Work out the finished part from the listing and answer in its coordinate system (mm). Coordinates: 2 decimals unless noted, no trailing zeros. Loops run counter-clockwise (first coordinate to the right, second up) from the corner with the lowest first, then second, coordinate; pieces in that order, holes last.
```python
from build123d import *

# Parameters (mm, degrees)
SKETCH1_R                                = 4.25
BOSS_EXTRUDE1_DEPTH                      = 10
BOSS_EXTRUDE2_START                      = -5
BOSS_EXTRUDE2_DEPTH                      = 15
SKETCH3_W                                = 342
SKETCH3_H                                = 10
BOSS_EXTRUDE3_DEPTH                      = 304
CUT_EXTRUDE1_REACH                       = 381.323
BOSS_EXTRUDE4_DEPTH                      = 3
MIRROR5_AT_THE_SECOND_PLANE_COPY_1_DEPTH = 3


with BuildPart() as part:
    # Sketch1 → Boss-Extrude1 (new body)
    with BuildSketch(Plane(origin=(0, 0, 0), x_dir=(1, 0, 0), z_dir=(0, 1, 0))):
        Polygon((-171, 11.25), (171, 11.25), (171, 0), (171, -13.75), (158, -13.75), (158, 0), (-158, 0), (-158, -13.75), (-171, -13.75), align=None)
        with Locations(Location((-164, 4.25, 0), (0, 0, 270))):
            Circle(SKETCH1_R, mode=Mode.SUBTRACT)
        with Locations(Location((164, 4.25, 0), (0, 0, 90))):
            Circle(SKETCH1_R, mode=Mode.SUBTRACT)
    boss_extrude1 = extrude(amount=BOSS_EXTRUDE1_DEPTH)

    # Sketch2 → Boss-Extrude2 (add)
    with BuildSketch(Plane.XY.offset(13.75).offset(BOSS_EXTRUDE2_START)):
        Polygon((-171, 85), (-171, 0), (-158, 0), (-158, 60), (158, 60), (158, 0), (171, 0), (171, 85), align=None)
    boss_extrude2 = extrude(amount=BOSS_EXTRUDE2_DEPTH)

    # Sketch3 → Boss-Extrude3 (add)
    with BuildSketch(Plane.XY.offset(23.75)):
        with Locations((0, 65)):
            Rectangle(SKETCH3_W, SKETCH3_H)
    extrude(amount=BOSS_EXTRUDE3_DEPTH)

    # Sketch4 → Cut-Extrude1 (cut, up to next)
    with BuildSketch(Plane(origin=(0, 85, 0), x_dir=(1, 0, 0), z_dir=(0, 1, 0)), mode=Mode.PRIVATE) as cut_extrude1_sk1:
        Polygon((-163.5, -23.75), (-5, -23.75), (-5, -327.75), (-163.5, -327.75), (-163.5, -39.75), (-163.5, -34.75), align=None)
    cut_extrude1_tool1 = extrude(cut_extrude1_sk1.sketch, amount=-CUT_EXTRUDE1_REACH, mode=Mode.PRIVATE) & part.part
    # Sketch4 → Cut-Extrude1 (cut, up to next)
    with BuildSketch(Plane(origin=(0, 85, 0), x_dir=(1, 0, 0), z_dir=(0, 1, 0)), mode=Mode.PRIVATE) as cut_extrude1_sk2:
        Polygon((163.5, -23.75), (163.5, -51.4723011), (163.5, -327.75), (5, -327.75), (5, -39.75), (5, -23.75), align=None)
    cut_extrude1_tool2 = extrude(cut_extrude1_sk2.sketch, amount=-CUT_EXTRUDE1_REACH, mode=Mode.PRIVATE) & part.part
    add(cut_extrude1_tool1.solids().sort_by_distance((-84.25, 85, 175.75))[0], mode=Mode.SUBTRACT)
    add(cut_extrude1_tool2.solids().sort_by_distance((84.25, 85, 175.75))[0], mode=Mode.SUBTRACT)

    # Mirror3: Boss-Extrude2 across plane
    add(boss_extrude2.mirror(Plane(origin=(0, 0, 175.75), x_dir=(1, 0, 0), z_dir=(0, 0, -1))))

    # Mirror4: Boss-Extrude1 across plane
    add(boss_extrude1.mirror(Plane(origin=(0, 0, 175.75), x_dir=(1, 0, 0), z_dir=(0, 0, -1))))

    # Sketch7 → Boss-Extrude4 (add)
    with BuildSketch(Plane(origin=(0, 60, 0), x_dir=(-1, 0, 0), z_dir=(0, -1, 0))):
        Polygon((-163.5, -23.75), (-148.5, -23.75), (-163.5, -38.75), align=None)
        Polygon((-5, -23.75), (-20, -23.75), (-5, -38.75), align=None)
    boss_extrude4 = extrude(amount=-BOSS_EXTRUDE4_DEPTH)

    # Mirror5: Boss-Extrude4 across plane
    add(boss_extrude4.mirror(Plane(origin=(0, 0, 175.75), x_dir=(1, 0, 0), z_dir=(0, 0, -1))))

    # Mirror5 at the second plane: Boss-Extrude4 across plane
    add(boss_extrude4.mirror(Plane(origin=(0, 0, 0), x_dir=(0, 0, 1), z_dir=(1, 0, 0))))

    # Mirror5 at the second plane copy 1 sketc → Mirror5 at the second plane copy 1 (add)
    with BuildSketch(Plane(origin=(0, 60, 351.5), x_dir=(1, 0, 0), z_dir=(0, -1, 0))):
        Polygon((-163.5, -23.75), (-148.5, -23.75), (-163.5, -38.75), align=None)
        Polygon((-5, -23.75), (-20, -23.75), (-5, -38.75), align=None)
    extrude(amount=-MIRROR5_AT_THE_SECOND_PLANE_COPY_1_DEPTH)


solid = part.part
```
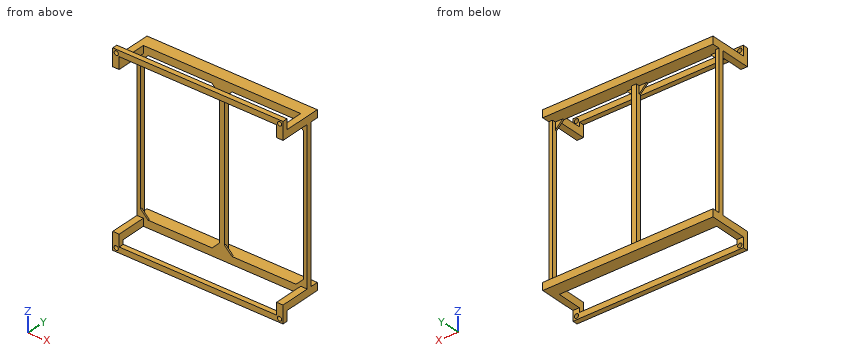
1. A cutting plane is placed at B-B, the plane x = -36.5. Give the vertices of the cut face in (y, z), then the cut area to 3 significant figures.
2. A cutting plane is placed at A-A, the plane z = 47. Give the vertices of the cut face in (x, y), then the cut area to 3 significant figures.
3. Straight lines are drawn through the part: probe 1 along X at (y, z) = (65.5, 43); probe 2 along X at (y, z) = (2, 355); probe 3 along Z at (x, y) = (164, 3.75). For each, find the intervals that lie inside material, in ascending order.
4. A cutting plane is placed at C-C, the plane z = -4.25. Give the vertices of the cut face in (x, y).
5. Each of these flat-tipped pins is pushed along its axis until it touches: P1, Ø7.5, axis at x = 10, z = 317, coming from the +Y side; P2, Ø12, axis at y = 72.5, z = 162, coming from the -X side; P3, Ø2, axis at x = -168.5, z = 151, coming from the +Y side; P4, Ø10.5, axis at x = 167, y = 17, coming from the +Z side. Where does it stop, or does it pass through?
Answers below:
1. outline: (0, -11.25) - (10, -11.25) - (10, 0) - (0, 0) - close; (0, 351.5) - (10, 351.5) - (10, 362.75) - (0, 362.75) - close; (60, 8.75) - (85, 8.75) - (85, 23.75) - (60, 23.75) - close; (60, 327.75) - (85, 327.75) - (85, 342.75) - (60, 342.75) - close
1. area: 975 mm2
2. outline: (-171, 60) - (-163.5, 60) - (-163.5, 70) - (-171, 70) - close; (-5, 60) - (5, 60) - (5, 70) - (-5, 70) - close; (163.5, 60) - (171, 60) - (171, 70) - (163.5, 70) - close
2. area: 250 mm2
3. probe 1: x = -171 to -163.5, -5 to 5, 163.5 to 171
3. probe 2: x = -171 to -168.18, -159.82 to 159.82, 168.18 to 171
3. probe 3: z = -11.25 to -8.5, 0 to 23.75, 327.75 to 351.5, 360 to 362.75
4. outline: (-171, 0) - (-168.25, 0) - (-168.25, 10) - (-171, 10) - close; (-159.75, 0) - (159.75, 0) - (159.75, 10) - (-159.75, 10) - close; (168.25, 0) - (171, 0) - (171, 10) - (168.25, 10) - close
5. P1: stops at y = 63
5. P2: stops at x = -171
5. P3: stops at y = 70
5. P4: stops at z = 342.75
